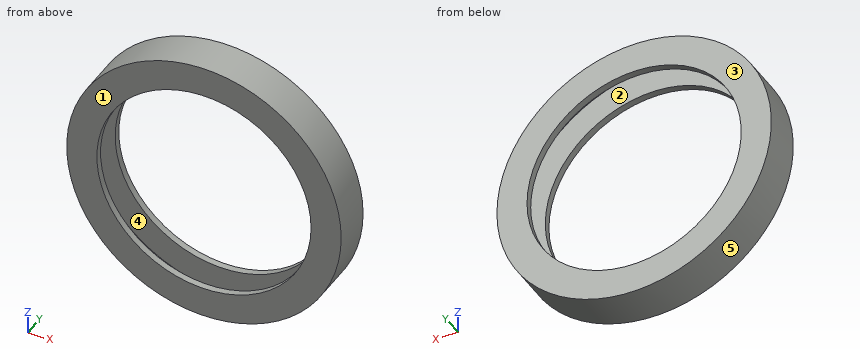
from build123d import *

# Parameters (mm, degrees)
F0_R     = 20.5
F0_R_2   = 20
F1_DEPTH = 6
F0_R_3   = 16
F2_DEPTH = 1
F3_R     = 20
F3_R_2   = 16
F4_DEPTH = 1


with BuildPart() as f1:
    # F0 (on Front) → F1 (new body)
    with BuildSketch(Plane.XZ):
        Circle(F0_R)
        Circle(F0_R_2, mode=Mode.SUBTRACT)
    extrude(amount=F1_DEPTH)

    # F0 (on Front) → F2 (join)
    with BuildSketch(Plane.XZ):
        Circle(F0_R_2)
        Circle(F0_R_3, mode=Mode.SUBTRACT)
    extrude(amount=F2_DEPTH)

    # F3 (on face) → F4 (join)
    with BuildSketch(Plane.XZ.offset(6)):
        Circle(F3_R)
        Circle(F3_R_2, mode=Mode.SUBTRACT)
    extrude(amount=-F4_DEPTH)


solid = f1.part
Part model, mm, in its own coordinate system. Face numbers are marked on the shaded views. A direction names the side the tool comes from. Coordinates: 2 decimals unless noted, no trailing zeros. Write each loop counter-clockwise with the first axis right and the second up, starting at its lowest first coordinate (ties: lowest second). Pieces come first, ordered by that corner, then holes. Notation, with made-up numbers: M 62,46 L 68,46 A30 ccw 68,70 Z; hole C 41,1.25 d1. An arc over 180 degrees is marked long. Return JSON: item names as keys, results as strings.
1. Probe L1, parallel to Y at x = 14, z = -9; L2, parallel to Z at x = 0, y = -2.6; L3, parallel to Z at x = 0, y = -0.65. List the from-to ranges inside material, lowest first.
Determined:
{"L1": "-6 to -5, -1 to 0", "L2": "-20.5 to -20, 20 to 20.5", "L3": "-20.5 to -16, 16 to 20.5"}
2. Pull direction X, two halves, no side cores. Call the marked faces 3, 4 and 5: pulls with the +X half, pulls with the -X half, needs draft (parallel to the pull), parting line crosses it, or undercut.
Determined:
{"face 3": "needs draft", "face 4": "undercut", "face 5": "parting line crosses it"}
3. Flat gauge pins, fed straight in: pin 1 Ø1.5 at (y, z) = (-4.5, -6.5) entering from -X; pin 2 Ø3 at (x, y) = (15.5, -5) entering from -Z (3 decimals); pin 3 Ø2 at (x, y) = (-8.5, -2.5) entering from +Z. Where does each tip first touch, or does it go through?
Determined:
{"pin 1": "x = -19.68", "pin 2": "z = -14.975", "pin 3": "z = 19.08"}
4. Saw through at A-A, the plane x = 0. Write the cut outline in (y, z), then the cut area to 3 significant figures.
Determined:
{"outline": "M -6,-20.5 L 0,-20.5 L 0,-16 L -1,-16 L -1,-20 L -5,-20 L -5,-16 L -6,-16 Z; M -6,16 L -5,16 L -5,20 L -1,20 L -1,16 L 0,16 L 0,20.5 L -6,20.5 Z", "area": "22.0 mm²"}
5. 3-axis set-ups, long thin cutter, end or side, ignore diameter. For the marked faces 1 and 2: which of +Z, -Z, +X, -X, +Y, -Y reach the whole face in a straight line?
Determined:
{"face 1": "+Z, -Z, +X, -X, -Y", "face 2": "none"}
6. Saw through at B-B, the plane z = 0. Write the cut outline in (x, y).
Determined:
{"outline": "M -20.5,-6 L -16,-6 L -16,-5 L -20,-5 L -20,-1 L -16,-1 L -16,0 L -20.5,0 Z; M 16,-6 L 20.5,-6 L 20.5,0 L 16,0 L 16,-1 L 20,-1 L 20,-5 L 16,-5 Z"}
7. Saw through at C-C, the plane y = -2.65. Write the cut outline in (x, z), then the cut area to 3 significant figures.
Determined:
{"outline": "C 0,0 d41; hole C 0,0 d40", "area": "63.6 mm²"}
